```python
from build123d import *

# Parameters (mm, degrees)
F0_R     = 298.45
F0_R_2   = 292.1
F0_R_3   = 285.75
F1_DEPTH = 12.7
F2_DEPTH = 876.3
F3_R     = 298.45
F4_DEPTH = 12.7


with BuildPart() as f1:
    # F0 (on Top) → F1 (new body)
    with BuildSketch(Plane.XY):
        Circle(F0_R)
        Circle(F0_R_2, mode=Mode.SUBTRACT)
        Circle(F0_R_2)
        Circle(F0_R_3, mode=Mode.SUBTRACT)
        Circle(F0_R_3)
    extrude(amount=F1_DEPTH)

    # F0 (on Top) → F2 (join)
    with BuildSketch(Plane.XY):
        Circle(F0_R_2)
        Circle(F0_R_3, mode=Mode.SUBTRACT)
    extrude(amount=F2_DEPTH)

    # F3 (on face) → F4 (join)
    with BuildSketch(Plane.XY.offset(876.3)):
        Circle(F3_R)
    extrude(amount=-F4_DEPTH)


solid = f1.part
```
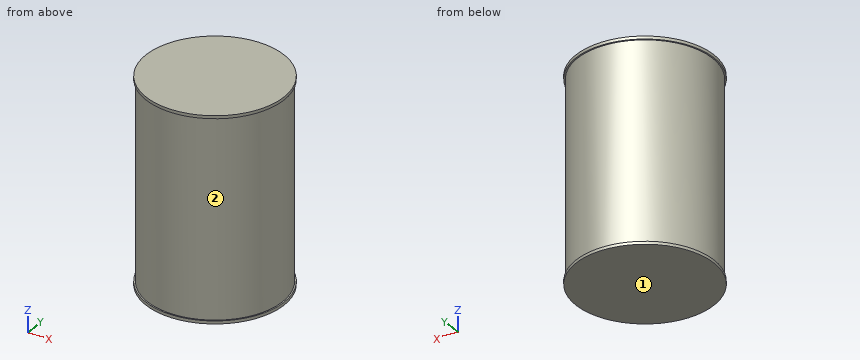
Read the model definition and answer for the solid it produces. Units are mm, in the model's axes. Face numbers are marked on the shaded views. A direction names the side the tool comes from. Give positions to 0.01 mm unless a question says otherwise; leave off trailing zeros. Order: outer loops, then holes, each group sorted by start corner. A loop starts at its lowest first (then second) coordinate and runs counter-clockwise, first axis right, second up.
(1) Straight lines are drawn through the part: L1, parallel to Z at x = 227.5, y = 119; L2, parallel to Y at x = 0, z = 618. For each, find the intervals that lie inside material, in ascending order.
(2) Find section C-C (z = 177.5). Give the vertices of the cut face in (x, y).
(3) Given pin 1 (4 mm diameter, centred on x = 116.5, z = 462.5, fed in from +Y); pin 2 (6 mm diameter, centred on x = 55.5, z = 699, fed in from -Y); pin 3 (2 mm diameter, centred on x = -238, z = 439.5, fed in from -Y); pin 4 (1.5 mm diameter, centred on x = -5.5, y = -194, fed in from -Z), each flat-ended and moving along its own axis, determine where each tip first touches the part or whether it passes through.
(4) Find section A-A (x = -88). Give the vertices of the cut face in (y, z), plus the area to 3 significant figures.
(5) Find section B-B (y = -226). Give the vertices of the cut face in (x, z).
(6) For the marked faces 1 and 2, determine the directions among +Z, -Z, +X, -X, +Y, -Y from which every point of the face is accessible in a straight line to the end or side of a thin tool.
Result sheet:
1. L1: z = 0 to 12.7, 863.6 to 876.3
1. L2: y = -292.1 to -285.75, 285.75 to 292.1
2. outline: circle Ø584.2 at (0, 0); hole circle Ø571.5 at (0, 0)
3. pin 1: stops at y = 268.72
3. pin 2: stops at y = -287.34
3. pin 3: stops at y = -170.74
3. pin 4: stops at z = 0
4. outline: (-285.18, 0) - (285.18, 0) - (285.18, 12.7) - (278.53, 12.7) - (278.53, 863.6) - (285.18, 863.6) - (285.18, 876.3) - (-285.18, 876.3) - (-285.18, 863.6) - (-278.53, 863.6) - (-278.53, 12.7) - (-285.18, 12.7) - close; hole (-271.86, 12.7) - (271.86, 12.7) - (271.86, 863.6) - (-271.86, 863.6) - close
4. area: 25,800 mm2
5. outline: (-194.93, 0) - (194.93, 0) - (194.93, 12.7) - (185.06, 12.7) - (185.06, 863.6) - (194.93, 863.6) - (194.93, 876.3) - (-194.93, 876.3) - (-194.93, 863.6) - (-185.06, 863.6) - (-185.06, 12.7) - (-194.93, 12.7) - close; hole (-174.86, 12.7) - (174.86, 12.7) - (174.86, 863.6) - (-174.86, 863.6) - close
6. face 1: -Z, +X, -X, +Y, -Y
6. face 2: none
